```python
from build123d import *

# Parameters (mm, degrees)
F0_R     = 1.524
F1_DEPTH = 6.35
F2_R     = 1.651
F3_DEPTH = 6.351
F4_R     = 1.778
F5_DEPTH = 6.351
F6_W     = 10
F6_H     = 50
F6_W_2   = 9
F6_H_2   = 21
F6_R     = 1
F7_DEPTH = 6.351


with BuildPart() as f1:
    # F0 (on Top) → F1 (new body)
    with BuildSketch(Plane.XY):
        with BuildLine():
            Line((36.191804, 81.707741), (-65.408196, 81.707741))
            ThreePointArc((-65.408196, 81.707741), (-83.368708, 74.268254), (-90.808196, 56.307741))
            Line((-90.808196, 56.307741), (-90.808196, -19.892259))
            ThreePointArc((-90.808196, -19.892259), (-68.489733, -73.773795), (-14.608196, -96.092259))
            ThreePointArc((-14.608196, -96.092259), (39.273341, -73.773795), (61.591804, -19.892259))
            Line((61.591804, -19.892259), (61.591804, 56.307741))
            ThreePointArc((61.591804, 56.307741), (54.152316, 74.268254), (36.191804, 81.707741))
        make_face()
        with Locations((-42.108196, -53.292259)):
            Circle(F0_R, mode=Mode.SUBTRACT)
        with Locations((12.891804, -53.292259)):
            Circle(F0_R, mode=Mode.SUBTRACT)
        with Locations((-42.108196, 31.707741)):
            Circle(F0_R, mode=Mode.SUBTRACT)
        with Locations((12.891804, 31.707741)):
            Circle(F0_R, mode=Mode.SUBTRACT)
    extrude(amount=F1_DEPTH)

    # F2 (on face) → F3 (cut, through all)
    with BuildSketch(Plane.XY.offset(6.35)):
        with Locations((-80.808196, 66.707741)):
            Circle(F2_R)
        with Locations((-80.808196, 45.007741)):
            Circle(F2_R)
        with Locations((-55.408196, 66.707741)):
            Circle(F2_R)
        with Locations((-55.408196, 45.007741)):
            Circle(F2_R)
        with Locations((26.191804, 66.707741)):
            Circle(F2_R)
        with Locations((51.591804, 66.707741)):
            Circle(F2_R)
        with Locations((26.191804, 45.007741)):
            Circle(F2_R)
        with Locations((51.591804, 45.007741)):
            Circle(F2_R)
    extrude(amount=-F3_DEPTH, mode=Mode.SUBTRACT)

    # F4 (on face) → F5 (cut, through all)
    with BuildSketch(Plane.XY.offset(6.35)):
        with Locations((-14.608196, -86.092259)):
            Circle(F4_R)
    extrude(amount=-F5_DEPTH, mode=Mode.SUBTRACT)

    # F6 (on face) → F7 (cut, through all)
    with BuildSketch(Plane.XY.offset(6.35)):
        with Locations((-60.808196, -26.092259)):
            Rectangle(F6_W, F6_H)
        with Locations((31.591804, -26.092259)):
            Rectangle(F6_W, F6_H)
        with Locations((-14.608196, 62.207741)):
            Rectangle(F6_W_2, F6_H_2)
        with Locations((-14.608196, 74.207741)):
            Circle(F6_R)
        with Locations((-14.608196, 50.207741)):
            Circle(F6_R)
    extrude(amount=-F7_DEPTH, mode=Mode.SUBTRACT)


solid = f1.part
```
Can you work these out from the model? Positions are in its coordinate system, mm. A direction names the side the tool comes from. Give positions to 0.01 mm unless a question says otherwise; leave off trailing zeros. Write each loop counter-clockwise with the first axis right and the second up, starting at its lowest first coordinate (ties: lowest second). Pieces come first, ordered by that corner, then holes. Notation, with made-up numbers: (41.25, -39.5) -> (80.25, -39.5) arc R10 ccw to (80.25, -21.5) -> close; hole circle Ø1 at (42.5, -35). An arc over 180 degrees is marked (long way). Write item = value, one per line.
(1) I need wall thicknesses on probe 1 along X at (y, z) = (-13.5, 1.75); probe 2 along Y at (x, z) = (-16, 3.5); probe 3 along X at (y, z) = (-24.5, 5.25). Which ranges of each line are inside material? Lowest first, please. Write a range as from..to.
Worked out:
probe_1 = -90.81..-65.81, -55.81..26.59, 36.59..61.59
probe_2 = -96.08..-87.2, -84.99..51.71, 72.71..81.71
probe_3 = -90.67..-65.81, -55.81..26.59, 36.59..61.45
(2) For faces 4 (the face through (-19.108, 62, 3)), 5 (the face through (-14, 81.708, 3)), which set-ups out of +Z, -Z, +X, -X, +Y, -Y let a thin tool reach every point of the face, with its end or its side?
Worked out:
face_4 = +Z, -Z
face_5 = +Z, -Z, +X, -X, +Y
(3) Thinking about a two-plate mould opening in Y: for faces 1 (the face through (54.35, 74.07, 3.13)), 2 (the face through (-90.808, 19, 3)), 3 (the face through (-16, -87.2, 3.2)), which applies, released by +Y, released by -Y, zero draft, split by the parting line, or undercut?
Worked out:
face_1 = released by +Y
face_2 = zero draft
face_3 = undercut
(4) I'm going to push flat-ended pins straight in: P1, Ø2.5, axis at x = 51.59, y = 45.01, coming from the +Z side; P2, Ø3, axis at y = -34.5, z = 3, coming from the -X side; P3, Ø1, axis at y = -47, z = 4, coming from the -X side. Where does each tip first touch, or does it pass through?
Worked out:
P1 = through
P2 = -89.67
P3 = -86.01
(5) Suppose I cut it at D-D on z = 5. Count the separate pieces of the cut face and the enclosed holes in it, then the cut area to 3 significant figures.
Worked out:
separate_pieces = 1
enclosed_holes = 18
area = 23,000 mm^2
(6) Suppose I cut it at A-A on y = -13.5. Write out the boundary of the cut face in (x, z).
Worked out:
outline = (-90.81, 0) -> (-65.81, 0) -> (-65.81, 6.35) -> (-90.81, 6.35) -> close; (-55.81, 0) -> (26.59, 0) -> (26.59, 6.35) -> (-55.81, 6.35) -> close; (36.59, 0) -> (61.59, 0) -> (61.59, 6.35) -> (36.59, 6.35) -> close
(7) Suppose I cut it at B-B on x = -63.5. Write out the boundary of the cut face in (y, z), then the cut area to 3 significant figures.
Worked out:
outline = (-78.34, 0) -> (-51.09, 0) -> (-51.09, 6.35) -> (-78.34, 6.35) -> close; (-1.09, 0) -> (81.71, 0) -> (81.71, 6.35) -> (-1.09, 6.35) -> close
area = 699 mm^2
(8) Suppose I cut it at C-C on y = 54. Write out the boundary of the cut face in (x, z).
Worked out:
outline = (-90.81, 0) -> (-19.11, 0) -> (-19.11, 6.35) -> (-90.81, 6.35) -> close; (-10.11, 0) -> (61.59, 0) -> (61.59, 6.35) -> (-10.11, 6.35) -> close
